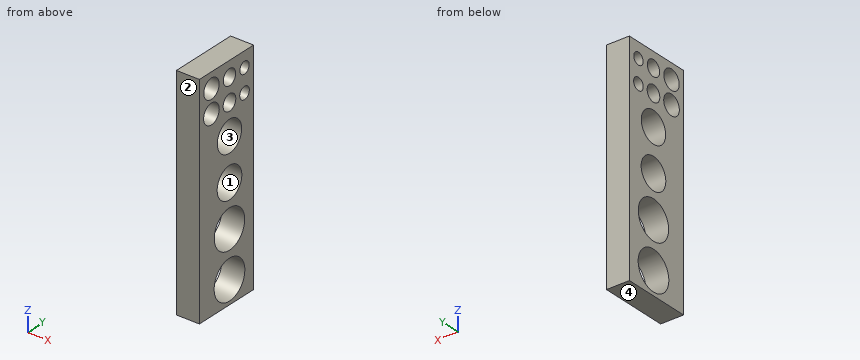
from build123d import *

# Parameters (mm, degrees)
SKETCH_1_W      = 58
SKETCH_1_H      = 18
SKETCH_1_R      = 2.05
SKETCH_1_R_2    = 2.1
SKETCH_1_R_3    = 1.55
SKETCH_1_R_4    = 1.6
SKETCH_1_R_5    = 2.55
SKETCH_1_R_6    = 2.6
SKETCH_1_R_7    = 4.05
SKETCH_1_R_8    = 4.1
SKETCH_1_R_9    = 5.05
SKETCH_1_R_10   = 5.1
EXTRUDE_1_DEPTH = 6


with BuildPart() as part:
    # 草图1 → 凸台-拉伸1 (new body)
    with BuildSketch(Plane(origin=(0, 0, 0), x_dir=(0, 0, -1), z_dir=(1, 0, 0))):
        with Locations((25, -1)):
            Rectangle(SKETCH_1_W, SKETCH_1_H)
        Circle(SKETCH_1_R, mode=Mode.SUBTRACT)
        with Locations((6, 0)):
            Circle(SKETCH_1_R_2, mode=Mode.SUBTRACT)
        with Locations((0, 5)):
            Circle(SKETCH_1_R_3, mode=Mode.SUBTRACT)
        with Locations((6, 5)):
            Circle(SKETCH_1_R_4, mode=Mode.SUBTRACT)
        with Locations((0, -6)):
            Circle(SKETCH_1_R_5, mode=Mode.SUBTRACT)
        with Locations((6, -6)):
            Circle(SKETCH_1_R_6, mode=Mode.SUBTRACT)
        with Locations((14, 0)):
            Circle(SKETCH_1_R_7, mode=Mode.SUBTRACT)
        with Locations((25, 0)):
            Circle(SKETCH_1_R_8, mode=Mode.SUBTRACT)
        with Locations((36, 0)):
            Circle(SKETCH_1_R_9, mode=Mode.SUBTRACT)
        with Locations((48, 0)):
            Circle(SKETCH_1_R_10, mode=Mode.SUBTRACT)
    extrude(amount=EXTRUDE_1_DEPTH)


solid = part.part
Verification items for the finished model (mm, model axes). Face numbers are marked on the shaded views. Coordinates: 2 decimals unless noted, no trailing zeros. Order: outer loops, then holes, each group sorted by start corner. A loop starts at its lowest first (then second) coordinate and runs counter-clockwise, first axis right, second up.
Item 1: Material ranges on L1, parallel to Y at x = 1.8, z = -6; L2, parallel to Y at x = 1.9, z = 0; L3, parallel to Z at x = 1.9, y = -7.5, recorded low to high.
Filled in:
L1: y = -10 to -8.6, -3.4 to -2.1, 2.1 to 3.4, 6.6 to 8
L2: y = -10 to -8.55, -3.45 to -2.05, 2.05 to 3.45, 6.55 to 8
L3: z = -54 to -8.12, -3.88 to -2.06, 2.06 to 4
Item 2: Section check C-C, the plane z = -37. Enter the section's corners in (x, y).
Filled in:
outline: (0, -10) - (6, -10) - (6, -4.95) - (0, -4.95) - close; (0, 4.95) - (6, 4.95) - (6, 8) - (0, 8) - close
Item 3: Release check for a two-part mould opening along Y. For the marked faces 1, 2, 3 and 4 record: +Y half, -Y half, draft (parallel to the pull), parting line (faces both ways), or undercut.
Filled in:
face 1: undercut
face 2: -Y half
face 3: undercut
face 4: draft
Item 4: Section check A-A, the plane z = 0. Enter the section's corners in (x, y), then the cut area to 3 significant figures.
Filled in:
outline: (0, -10) - (6, -10) - (6, -8.55) - (0, -8.55) - close; (0, -3.45) - (6, -3.45) - (6, -2.05) - (0, -2.05) - close; (0, 2.05) - (6, 2.05) - (6, 3.45) - (0, 3.45) - close; (0, 6.55) - (6, 6.55) - (6, 8) - (0, 8) - close
area: 34.2 mm2
Item 5: Section check D-D, the plane y = -7.75. Enter the section's corners in (x, z).
Filled in:
outline: (0, -54) - (6, -54) - (6, -7.92) - (0, -7.92) - close; (0, -4.08) - (6, -4.08) - (6, -1.85) - (0, -1.85) - close; (0, 1.85) - (6, 1.85) - (6, 4) - (0, 4) - close
Item 6: Section check B-B, the plane x = 2.5. Give the number of separate pieces and of enclosed holes in the cut face, then the cut area to 3 significant figures.
Filled in:
separate pieces: 1
enclosed holes: 10
area: 694 mm2
